Geometry: final body of the model. Coordinates: model frame, mm. Face numbers are marked on the shaded views. Round coordinates to 2 decimals unless told otherwise and drop trailing zeros. Loops run counter-clockwise (first coordinate to the right, second up) from the corner with the lowest first, then second, coordinate; pieces in that order, holes last. Notation, with made-up numbers: (69, 44.5) - (76, 44.5) arc R4 ccw to (76, 50.5) - close; hole circle Ø11 at (-12, 27). An arc over 180 degrees is marked (long way). Use CSV: the item, a comma, the result in double quotes.
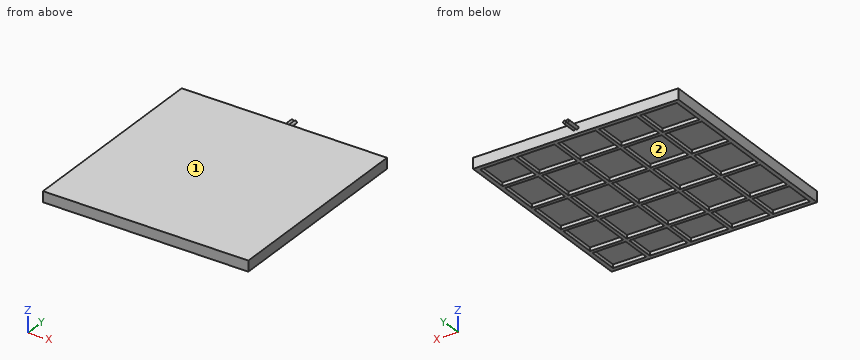
from build123d import *

# Parameters (mm, degrees)
ESQUISSE1_W        = 145
ESQUISSE1_H        = 145
BOSS_EXTRU_1_DEPTH = 5
ESQUISSE2_W        = 26.5
ESQUISSE2_H        = 28
BOSS_EXTRU_2_DEPTH = 2.5
ESQUISSE3_W        = 145
ESQUISSE3_H        = 145
ESQUISSE3_W_2      = 139
ESQUISSE3_H_2      = 139
BOSS_EXTRU_3_DEPTH = 2.5
ESQUISSE4_R        = 1
BOSS_EXTRU_4_DEPTH = 10


with BuildPart() as part:
    # Esquisse1 → Boss.-Extru.1 (new body)
    with BuildSketch(Plane.XY):
        Rectangle(ESQUISSE1_W, ESQUISSE1_H)
    extrude(amount=BOSS_EXTRU_1_DEPTH)

    # Esquisse2 → Boss.-Extru.2 (add)
    with BuildSketch(Plane(origin=(0, 0, 0), x_dir=(-1, 0, 0), z_dir=(0, 0, -1))):
        Polygon((-14.5, -48), (12, -48), (12, -72.5), (14.5, -72.5), (14.5, -48), (41, -48), (41, -72.5), (43.5, -72.5), (43.5, -48), (72.5, -48), (72.5, -45.5), (43.5, -45.5), (43.5, -17.5), (72.5, -17.5), (72.5, -15), (43.5, -15), (43.5, 13), (72.5, 13), (72.5, 15.5), (43.5, 15.5), (43.5, 43.5), (72.5, 43.5), (72.5, 46), (43.5, 46), (43.5, 72.5), (41, 72.5), (41, 46), (14.5, 46), (14.5, 72.5), (12, 72.5), (12, 46), (-14.5, 46), (-14.5, 72.5), (-17, 72.5), (-17, 46), (-43.5, 46), (-43.5, 72.5), (-46, 72.5), (-46, 46), (-72.5, 46), (-72.5, 43.5), (-46, 43.5), (-46, 15.5), (-72.5, 15.5), (-72.5, 13), (-46, 13), (-46, -15), (-72.5, -15), (-72.5, -17.5), (-46, -17.5), (-46, -45.5), (-72.5, -45.5), (-72.5, -48), (-46, -48), (-46, -72.5), (-43.5, -72.5), (-43.5, -48), (-17, -48), (-17, -72.5), (-14.5, -72.5), align=None)
        with Locations((27.75, -31.5)):
            Rectangle(ESQUISSE2_W, ESQUISSE2_H, mode=Mode.SUBTRACT)
        with Locations((-30.25, -31.5)):
            Rectangle(ESQUISSE2_W, ESQUISSE2_H, mode=Mode.SUBTRACT)
        with Locations((-1.25, -31.5)):
            Rectangle(ESQUISSE2_W, ESQUISSE2_H, mode=Mode.SUBTRACT)
        with Locations((-30.25, -1)):
            Rectangle(ESQUISSE2_W, ESQUISSE2_H, mode=Mode.SUBTRACT)
        with Locations((-30.25, 29.5)):
            Rectangle(ESQUISSE2_W, ESQUISSE2_H, mode=Mode.SUBTRACT)
        with Locations((-1.25, -1)):
            Rectangle(ESQUISSE2_W, ESQUISSE2_H, mode=Mode.SUBTRACT)
        with Locations((27.75, -1)):
            Rectangle(ESQUISSE2_W, ESQUISSE2_H, mode=Mode.SUBTRACT)
        with Locations((-1.25, 29.5)):
            Rectangle(ESQUISSE2_W, ESQUISSE2_H, mode=Mode.SUBTRACT)
        with Locations((27.75, 29.5)):
            Rectangle(ESQUISSE2_W, ESQUISSE2_H, mode=Mode.SUBTRACT)
    extrude(amount=BOSS_EXTRU_2_DEPTH)

    # Esquisse3 → Boss.-Extru.3 (add)
    with BuildSketch(Plane(origin=(0, 0, 0), x_dir=(-1, 0, 0), z_dir=(0, 0, -1))):
        Rectangle(ESQUISSE3_W, ESQUISSE3_H)
        Rectangle(ESQUISSE3_W_2, ESQUISSE3_H_2, mode=Mode.SUBTRACT)
    extrude(amount=BOSS_EXTRU_3_DEPTH)

    # Esquisse4 → Boss.-Extru.4 (add)
    with BuildSketch(Plane(origin=(0, 72.5, 0), x_dir=(1, 0, 0), z_dir=(0, 1, 0))):
        with Locations(Location((-1.1, -1.25, 0), (0, 0, 90))):
            Circle(ESQUISSE4_R)
        with Locations(Location((1.1, -1.25, 0), (0, 0, 90))):
            Circle(ESQUISSE4_R)
    extrude(amount=BOSS_EXTRU_4_DEPTH)


solid = part.part
Item 1: Pin query (flat end, axial travel): P1, Ø1.2, axis at x = 27, z = -1.5, coming from the +Y side; P2, Ø12, axis at x = -53.5, y = 6.5, coming from the -Z side. Return the tip coordinate at first contact, or that it passes through.
Final values:
P1,"stops at y = 72.5"
P2,"stops at z = 0"
Item 2: Section B-B on y = -21. Return the cut outline in (x, z).
Final values:
outline,"(-72.5, -2.5) - (-69.5, -2.5) - (-69.5, 0) - (-43.5, 0) - (-43.5, -2.5) - (-41, -2.5) - (-41, 0) - (-14.5, 0) - (-14.5, -2.5) - (-12, -2.5) - (-12, 0) - (14.5, 0) - (14.5, -2.5) - (17, -2.5) - (17, 0) - (43.5, 0) - (43.5, -2.5) - (46, -2.5) - (46, 0) - (69.5, 0) - (69.5, -2.5) - (72.5, -2.5) - (72.5, 5) - (-72.5, 5) - close"
Item 3: Section A-A on x = 9. Return the cut outline in (y, z).
Final values:
outline,"(-72.5, -2.5) - (-69.5, -2.5) - (-69.5, 0) - (-48, 0) - (-48, -2.5) - (-45.5, -2.5) - (-45.5, 0) - (-17.5, 0) - (-17.5, -2.5) - (-15, -2.5) - (-15, 0) - (13, 0) - (13, -2.5) - (15.5, -2.5) - (15.5, 0) - (43.5, 0) - (43.5, -2.5) - (46, -2.5) - (46, 0) - (69.5, 0) - (69.5, -2.5) - (72.5, -2.5) - (72.5, 5) - (-72.5, 5) - close"
Item 4: Mould query, pull axis X, two halves, no side actions, for the marked faces 1 and 2. Classes: released by +X, released by -X, zero draft, split by the parting line, or undercut.
Final values:
face 1,"zero draft"
face 2,"undercut"
Item 5: Section C-C on z = -1.25. Give the number of separate pieces and of enclosed holes in the cut face, plus the area to 3 significant figures.
Final values:
separate pieces,"1"
enclosed holes,"25"
area,"4,380 mm²"
Item 6: Material intervals for line 1 (X direction, y = 11.5, z = -1.5); line 2 (Y direction, x = -23, z = -0.25); line 3 (Z direction, x = 0, y = 37), sorted ascending.
Final values:
line 1,"x = -72.5 to -69.5, -43.5 to -41, -14.5 to -12, 14.5 to 17, 43.5 to 46, 69.5 to 72.5"
line 2,"y = -72.5 to -69.5, -48 to -45.5, -17.5 to -15, 13 to 15.5, 43.5 to 46, 69.5 to 72.5"
line 3,"z = 0 to 5"
